Geometry: final body of the model. Coordinates: model frame, mm. A direction names the side the tool comes from. Round coordinates to 2 decimals unless told otherwise and drop trailing zeros. Write each loop counter-clockwise with the first axis right and the second up, starting at its lowest first coordinate (ties: lowest second). Pieces come first, ordered by that corner, then holes. Notation, with made-up numbers: M 23,2.25 L 42,2.25 A8 ccw 42,6.25 Z; hole C 11.5,-4.75 d9. An arc over 180 degrees is marked long. Use one line per item in the form item = value. Start each with the question number.
from build123d import *

# Parameters (mm, degrees)
EXTRUDE_3_DEPTH      = 5.5
EXTRUDE_4_DEPTH      = 6
EXTRUDE_4_DEPTH_BACK = 0.5
SKETCH_5_W           = 13
SKETCH_5_H           = 10
SKETCH_5_R           = 2.2
SKETCH_5_H_2         = 13.5
SKETCH_5_R_2         = 1.5


with BuildPart() as part:
    # Эскиз4 → Бобышка-Вытянуть3 (new body)
    with BuildSketch(Plane(origin=(0, 0, 0), x_dir=(1, 0, 0), z_dir=(0, 1, 0))):
        Polygon((-40.5, -48), (40.5, -48), (40.5, -35), (35, -35), (35, -25), (40.5, -25), (40.5, 21.5), (35, 21.5), (35, 35), (40.5, 35), (40.5, 48), (-40.5, 48), (-40.5, 35), (-35, 35), (-35, 16), (-40.5, 16), (-40.5, -25), (-35, -25), (-35, -35), (-40.5, -35), align=None)
    extrude(amount=EXTRUDE_3_DEPTH)

    # Эскиз5 → Бобышка-Вытянуть4 (add, two sides: drawn at the far end of the back side and taken through both)
    # profile 1 of 4: a face of its own
    with BuildSketch(Plane(origin=(0, 0, 0), x_dir=(1, 0, 0), z_dir=(0, 1, 0)).offset(-EXTRUDE_4_DEPTH_BACK)):
        with Locations((41.5, -30)):
            Rectangle(SKETCH_5_W, SKETCH_5_H)
        with Locations(Location((44, -30, 0), (0, 0, 270))):
            Circle(SKETCH_5_R, mode=Mode.SUBTRACT)
    # profile 2 of 4: a face of its own
    with BuildSketch(Plane(origin=(0, 0, 0), x_dir=(1, 0, 0), z_dir=(0, 1, 0)).offset(-EXTRUDE_4_DEPTH_BACK)):
        with Locations((-41.5, -30)):
            Rectangle(SKETCH_5_W, SKETCH_5_H)
        with Locations(Location((-44, -30, 0), (0, 0, 270))):
            Circle(SKETCH_5_R, mode=Mode.SUBTRACT)
    # profile 3 of 4: a face of its own
    with BuildSketch(Plane(origin=(0, 0, 0), x_dir=(1, 0, 0), z_dir=(0, 1, 0)).offset(-EXTRUDE_4_DEPTH_BACK)):
        with Locations((41.5, 28.25)):
            Rectangle(SKETCH_5_W, SKETCH_5_H_2)
        with Locations(Location((44, 30, 0), (0, 0, 270))):
            Circle(SKETCH_5_R, mode=Mode.SUBTRACT)
        with Locations(Location((43.5, 24, 0), (0, 0, 270))):
            Circle(SKETCH_5_R_2, mode=Mode.SUBTRACT)
    # profile 4 of 4: a face of its own
    with BuildSketch(Plane(origin=(0, 0, 0), x_dir=(1, 0, 0), z_dir=(0, 1, 0)).offset(-EXTRUDE_4_DEPTH_BACK)):
        Polygon((-48, 16), (-35, 16), (-35, 35), (-48, 35), (-48, 25.5), (-43, 25.5), (-43, 22.5), (-48, 22.5), align=None)
        with Locations(Location((-44, 30, 0), (0, 0, 270))):
            Circle(SKETCH_5_R, mode=Mode.SUBTRACT)
    extrude(amount=EXTRUDE_4_DEPTH + EXTRUDE_4_DEPTH_BACK)


solid = part.part
1. Section query C-C (y = 4.25). Give the number of separate pieces and of enclosed holes in the cut face, then the cut area to 3 significant figures.
2. Section query B-B (z = -24). Return loops of the section in (x, y), then the cut area to 3 significant figures.
3. Set-up query: faces 1 (the face through (-48, 3, -30)), 2 (the face through (-43, 3, -24)), 3 (the face through (-40.5, 3, -42)), 4 (the face through (40.5, 3, 42)). Return all of +Z, -Z, +X, -X, +Y, -Y with unobstructed straight access to the full face (end or side cutting, diameter ignored); none if empty.
4. Ray query, probe 1 along X at (y, z) = (3.25, 30); probe 2 along X at (y, z) = (1, -24); probe 3 along Y at (x, z) = (-1, 7). Return the intervals inside material, ascending.
5. Section query A-A (z = 30). Return loops of the section in (x, y).
6. Pull-direction query (X, two-part tool) for faces 5 (the face through (-40.5, 3, 41)), 6 (the face through (-41.6, -0.5, 29.9)), 7 (the face through (-1, 0, -1)); classes: released by +X, released by -X, zero draft, split by the parting line, or undercut.
7. Contact query for flat-ended pins moving along their axis: pin 1 (2 mm diameter, centred on x = -8.5, z = -32.5, fed in from +Y); pin 2 (2 mm diameter, centred on x = 44.5, y = 3, fed in from +Z); pin 3 (1.5 mm diameter, centred on y = 3.5, z = -11, fed in from +X); pin 4 (2.5 mm diameter, centred on x = 44, z = -30, fed in from -Y). Output: stop coordinate, or through.
8. Section query D-D (x = -12.5). Return loops of the section in (y, z), then the cut area to 3 significant figures.
Checks:
q1.separate_pieces = 1
q1.enclosed_holes = 5
q1.area = 8,090 mm^2
q2.outline = M -43,-0.5 L -35,-0.5 L -35,0 L 35,0 L 35,-0.5 L 42,-0.5 L 42,6 L 35,6 L 35,5.5 L -35,5.5 L -35,6 L -43,6 Z; M 45,-0.5 L 48,-0.5 L 48,6 L 45,6 Z
q2.area = 502 mm^2
q3.face_1 = +Z, -Z, -X, +Y, -Y
q3.face_2 = -X, +Y, -Y
q3.face_3 = -Z, -X, +Y, -Y
q3.face_4 = +Z, +X, +Y, -Y
q4.probe_1 = -48 to -46.2, -41.8 to 41.8, 46.2 to 48
q4.probe_2 = -43 to 42, 45 to 48
q4.probe_3 = 0 to 5.5
q5.outline = M -48,-0.5 L -46.2,-0.5 L -46.2,6 L -48,6 Z; M -41.8,-0.5 L -35,-0.5 L -35,0 L 35,0 L 35,-0.5 L 41.8,-0.5 L 41.8,6 L 35,6 L 35,5.5 L -35,5.5 L -35,6 L -41.8,6 Z; M 46.2,-0.5 L 48,-0.5 L 48,6 L 46.2,6 Z
q6.face_5 = released by -X
q6.face_6 = zero draft
q6.face_7 = undercut
q7.pin_1 = 5.5
q7.pin_2 = 35
q7.pin_3 = 40.5
q7.pin_4 = through
q8.outline = M 0,-48 L 5.5,-48 L 5.5,48 L 0,48 Z
q8.area = 528 mm^2
